Verification items for the finished model (mm, model axes). Face numbers are marked on the shaded views. Give positions to 0.01 mm unless a question says otherwise; leave off trailing zeros. Loops run counter-clockwise (first coordinate to the right, second up) from the corner with the lowest first, then second, coordinate; pieces in that order, holes last. Notation, with made-up numbers: M -11,16.25 L 8,16.25 A25 cw 8,40.25 Z; hole C 78,0.5 d3. An arc over 180 degrees is marked long. Answer in a Markdown table with one row per item.
```python
from build123d import *

# Parameters (mm, degrees)
ESBO_O1_W                  = 144
ESBO_O1_H                  = 74
ESBO_O1_W_2                = 140
ESBO_O1_H_2                = 70
RESSALTO_EXTRUS_O1_DEPTH   = 60
ESBO_O2_W                  = 144
ESBO_O2_H                  = 74
ESBO_O2_R                  = 2
RESSALTO_EXTRUS_O2_DEPTH   = 2
ESBO_O3_W                  = 14
ESBO_O3_H                  = 16
USB_FONTE_DEPTH            = 10
ESBO_O6_R                  = 1.65
ESBO_O6_W                  = 8
ESBO_O6_H                  = 35
SAIDA_DE_AR_DEPTH          = 1
SAIDA_DE_AR_DEPTH_BACK     = 75
ESBO_O7_W                  = 15
ESBO_O7_H                  = 30
DISPLAY_DEPTH              = 145
ESBO_O8_R                  = 4.5
ESBO_O8_R_2                = 1.35
RESSALTO_EXTRUS_O3_DEPTH   = 5
ESBO_O8_3_R                = 1.35
CORTE_EXTRUS_O4_DEPTH      = 3
ESBO_O9_R                  = 3
CORTE_EXTRUS_O5_DEPTH      = 2
CORTE_EXTRUS_O5_DEPTH_BACK = 10
RESSALTO_EXTRUS_O4_START   = -8
ESBO_O11_R                 = 1.65
RESSALTO_EXTRUS_O4_DEPTH   = 7
CORTE_EXTRUS_O6_DEPTH      = 3
ESBO_O13_R                 = 15.811388301
ESBO_O13_R_2               = 10
RESSALTO_EXTRUS_O5_DEPTH   = 2
ESBO_O13_3_R               = 10
CORTE_EXTRUS_O7_DEPTH      = 10
ESBO_O15_R                 = 22.5
ESBO_O15_R_2               = 1.6
CORTE_EXTRUS_O9_DEPTH      = 10
ESBO_O15_3_R               = 27.5
ESBO_O15_3_R_2             = 22.5
RESSALTO_EXTRUS_O6_DEPTH   = 2


with BuildPart() as part:
    # Esboço1 → Ressalto-extrusão1 (new body)
    with BuildSketch(Plane.XY):
        Rectangle(ESBO_O1_W, ESBO_O1_H)
        Rectangle(ESBO_O1_W_2, ESBO_O1_H_2, mode=Mode.SUBTRACT)
    extrude(amount=RESSALTO_EXTRUS_O1_DEPTH)

    # Esboço2 → Ressalto-extrusão2 (add)
    with BuildSketch(Plane(origin=(0, 0, 0), x_dir=(-1, 0, 0), z_dir=(0, 0, -1))):
        Rectangle(ESBO_O2_W, ESBO_O2_H)
        with Locations((-60, -27.5)):
            Circle(ESBO_O2_R, mode=Mode.SUBTRACT)
        with Locations((60, -27.5)):
            Circle(ESBO_O2_R, mode=Mode.SUBTRACT)
        with Locations((60, 27.5)):
            Circle(ESBO_O2_R, mode=Mode.SUBTRACT)
        with Locations((-60, 27.5)):
            Circle(ESBO_O2_R, mode=Mode.SUBTRACT)
    extrude(amount=-RESSALTO_EXTRUS_O2_DEPTH)

    # Esboço3 → USB + fonte (cut)
    with BuildSketch(Plane(origin=(72, 0, 0), x_dir=(0, 0, -1), z_dir=(1, 0, 0))):
        with Locations((-14, -17.1)):
            Rectangle(ESBO_O3_W, ESBO_O3_H)
    extrude(amount=-USB_FONTE_DEPTH, mode=Mode.SUBTRACT)

    # Esboço6 → saida de ar (cut, two sides)
    with BuildSketch(Plane.XZ.offset(37)) as saida_de_ar_sk:
        with Locations((-44, 50)):
            Circle(ESBO_O6_R)
        with Locations((44, 50)):
            Circle(ESBO_O6_R)
        with Locations((-58, 27.5)):
            Rectangle(ESBO_O6_W, ESBO_O6_H)
        with Locations((-45, 27.5)):
            Rectangle(ESBO_O6_W, ESBO_O6_H)
        with Locations((-32, 27.5)):
            Rectangle(ESBO_O6_W, ESBO_O6_H)
        with Locations((-19, 27.5)):
            Rectangle(ESBO_O6_W, ESBO_O6_H)
        with Locations((-6, 27.5)):
            Rectangle(ESBO_O6_W, ESBO_O6_H)
        with Locations((7, 27.5)):
            Rectangle(ESBO_O6_W, ESBO_O6_H)
        with Locations((20, 27.5)):
            Rectangle(ESBO_O6_W, ESBO_O6_H)
        with Locations((33, 27.5)):
            Rectangle(ESBO_O6_W, ESBO_O6_H)
        with Locations((46, 27.5)):
            Rectangle(ESBO_O6_W, ESBO_O6_H)
        with Locations((59, 27.5)):
            Rectangle(ESBO_O6_W, ESBO_O6_H)
    extrude(amount=SAIDA_DE_AR_DEPTH, mode=Mode.SUBTRACT)
    extrude(saida_de_ar_sk.sketch, amount=-SAIDA_DE_AR_DEPTH_BACK, mode=Mode.SUBTRACT)

    # Esboço7 → display (cut, through all)
    with BuildSketch(Plane.ZY.offset(72)):
        with Locations((52.5, 0)):
            Rectangle(ESBO_O7_W, ESBO_O7_H)
    extrude(amount=-DISPLAY_DEPTH, mode=Mode.SUBTRACT)

    # Esboço8 → Ressalto-extrusão3 (add)
    with BuildSketch(Plane(origin=(0, 0, 2), x_dir=(-1, 0, 0), z_dir=(0, 0, -1))):
        with Locations((32.3, 20.5)):
            Circle(ESBO_O8_R)
        with Locations((32.3, 20.5)):
            Circle(ESBO_O8_R_2, mode=Mode.SUBTRACT)
        with Locations((-50, 20.5)):
            Circle(ESBO_O8_R)
        with Locations((-50, 20.5)):
            Circle(ESBO_O8_R_2, mode=Mode.SUBTRACT)
        with Locations((-48.7, -27.67)):
            Circle(ESBO_O8_R)
        with Locations((-48.7, -27.67)):
            Circle(ESBO_O8_R_2, mode=Mode.SUBTRACT)
    extrude(amount=-RESSALTO_EXTRUS_O3_DEPTH)

    # Esboço8<3> → Corte-extrusão4 (cut, through all)
    with BuildSketch(Plane(origin=(0, 0, 2), x_dir=(-1, 0, 0), z_dir=(0, 0, -1))):
        with Locations((-48.7, -27.67)):
            Circle(ESBO_O8_3_R)
        with Locations((32.3, 20.5)):
            Circle(ESBO_O8_3_R)
        with Locations((-50, 20.5)):
            Circle(ESBO_O8_3_R)
    extrude(amount=CORTE_EXTRUS_O4_DEPTH, mode=Mode.SUBTRACT)

    # Esboço9 → Corte-extrusão5 (cut, two sides)
    with BuildSketch(Plane.XY.offset(2)) as corte_extrus_o5_sk:
        with Locations((50, 20.5)):
            Circle(ESBO_O9_R)
        with Locations((48.7, -27.67)):
            Circle(ESBO_O9_R)
        with Locations((-32.3, 20.5)):
            Circle(ESBO_O9_R)
    extrude(amount=CORTE_EXTRUS_O5_DEPTH, mode=Mode.SUBTRACT)
    extrude(corte_extrus_o5_sk.sketch, amount=-CORTE_EXTRUS_O5_DEPTH_BACK, mode=Mode.SUBTRACT)

    # Esboço11 → Ressalto-extrusão4 (add)
    with BuildSketch(Plane.XY.offset(60).offset(RESSALTO_EXTRUS_O4_START)):
        with BuildLine():
            Line((70, -25), (65, -25))
            ThreePointArc((65, -25), (60, -20), (65, -15))
            Line((65, -15), (70, -15))
            Line((70, -15), (70, -25))
        make_face()
        with Locations((65, -20)):
            Circle(ESBO_O11_R, mode=Mode.SUBTRACT)
        with BuildLine():
            Line((70, 35), (65, 35))
            ThreePointArc((65, 35), (61.464466094, 26.464466094), (70, 30))
            Line((70, 30), (70, 35))
        make_face()
        with Locations((65, 30)):
            Circle(ESBO_O11_R, mode=Mode.SUBTRACT)
        with BuildLine():
            Line((-70, -25), (-70, -15))
            Line((-70, -15), (-65, -15))
            ThreePointArc((-65, -15), (-60, -20), (-65, -25))
            Line((-65, -25), (-70, -25))
        make_face()
        with Locations((-65, -20)):
            Circle(ESBO_O11_R, mode=Mode.SUBTRACT)
        with BuildLine():
            Line((-65, 35), (-70, 35))
            Line((-70, 35), (-70, 30))
            ThreePointArc((-70, 30), (-61.464466094, 26.464466094), (-65, 35))
        make_face()
        with Locations((-65, 30)):
            Circle(ESBO_O11_R, mode=Mode.SUBTRACT)
    extrude(amount=-RESSALTO_EXTRUS_O4_DEPTH)

    # Esboço12 → Corte-extrusão6 (cut)
    with BuildSketch(Plane(origin=(0, 0, 45), x_dir=(-1, 0, 0), z_dir=(0, 0, -1))):
        Polygon((-61.824573519, 30), (-63.41228676, 32.75), (-66.58771324, 32.75), (-68.175426481, 30), (-66.58771324, 27.25), (-63.41228676, 27.25), align=None)
        Polygon((61.824573519, 30), (63.41228676, 27.25), (66.58771324, 27.25), (68.175426481, 30), (66.58771324, 32.75), (63.41228676, 32.75), align=None)
        Polygon((-61.824573519, -20), (-63.41228676, -17.25), (-66.58771324, -17.25), (-68.175426481, -20), (-66.58771324, -22.75), (-63.41228676, -22.75), align=None)
        Polygon((61.824573519, -20), (63.41228676, -22.75), (66.58771324, -22.75), (68.175426481, -20), (66.58771324, -17.25), (63.41228676, -17.25), align=None)
    extrude(amount=-CORTE_EXTRUS_O6_DEPTH, mode=Mode.SUBTRACT)

    # Esboço13 → Ressalto-extrusão5 (add)
    with BuildSketch(Plane(origin=(0, 37, 0), x_dir=(1, 0, 0), z_dir=(0, 1, 0))):
        with Locations((29, -25)):
            Circle(ESBO_O13_R)
        with Locations((29, -25)):
            Circle(ESBO_O13_R_2, mode=Mode.SUBTRACT)
    extrude(amount=-RESSALTO_EXTRUS_O5_DEPTH)

    # Esboço13<3> → Corte-extrusão7 (cut)
    with BuildSketch(Plane(origin=(0, 37, 0), x_dir=(1, 0, 0), z_dir=(0, 1, 0))):
        with Locations((29, -25)):
            Circle(ESBO_O13_3_R)
    extrude(amount=-CORTE_EXTRUS_O7_DEPTH, mode=Mode.SUBTRACT)

    # Esboço15 → Corte-extrusão9 (cut)
    with BuildSketch(Plane(origin=(0, 37, 0), x_dir=(1, 0, 0), z_dir=(0, 1, 0))):
        with Locations((-16, -31)):
            Circle(ESBO_O15_R)
        with Locations((-41, -56)):
            Circle(ESBO_O15_R_2)
        with Locations((9, -56)):
            Circle(ESBO_O15_R_2)
        with Locations((-41, -6)):
            Circle(ESBO_O15_R_2)
        with Locations((9, -6)):
            Circle(ESBO_O15_R_2)
    extrude(amount=-CORTE_EXTRUS_O9_DEPTH, mode=Mode.SUBTRACT)

    # Esboço15<3> → Ressalto-extrusão6 (add)
    with BuildSketch(Plane(origin=(0, 37, 0), x_dir=(1, 0, 0), z_dir=(0, 1, 0))):
        with Locations((-16, -31)):
            Circle(ESBO_O15_3_R)
        with Locations((-16, -31)):
            Circle(ESBO_O15_3_R_2, mode=Mode.SUBTRACT)
    extrude(amount=-RESSALTO_EXTRUS_O6_DEPTH)


solid = part.part
```
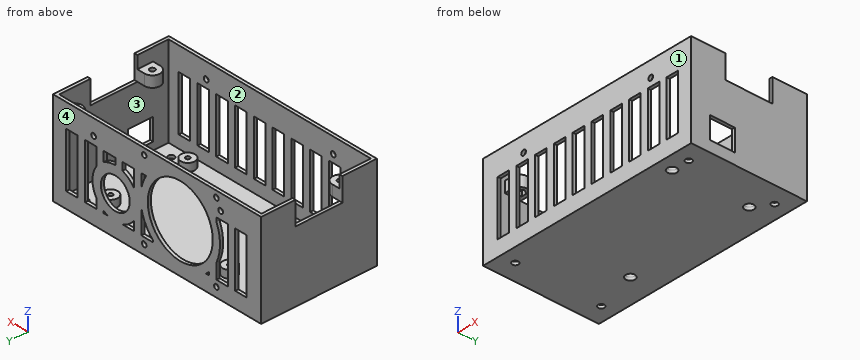
Item 1: Sectioned sample at C-C (y = 12.5). Record the cut outline in (x, z).
Reported:
| item | result |
|---|---|
| outline | M -72,0 L 72,0 L 72,45 L 70,45 L 70,2 L -70,2 L -70,45 L -72,45 Z |
Item 2: Release check for a two-part mould opening along Y. For the marked faces 1, 2, 3 and 4 record: released by +Y, released by -Y, zero draft, split by the parting line, or undercut.
Reported:
| item | result |
|---|---|
| face 1 | released by -Y |
| face 2 | undercut |
| face 3 | undercut |
| face 4 | released by +Y |
Item 3: Sectioned sample at B-B (x = 40.5). Record the cut outline in (y, z), and give its area (3 significant figures).
Reported:
| item | result |
|---|---|
| outline | M -37,0 L 37,0 L 37,60 L 35,60 L 35,2 L -35,2 L -35,60 L -37,60 Z |
| area | 380 mm^2 |
Item 4: Sectioned sample at A-A (y = -12.5). Record the cut outline in (x, z), and give its area (3 significant figures).
Reported:
| item | result |
|---|---|
| outline | M -72,0 L 72,0 L 72,7 L 70,7 L 70,2 L -70,2 L -70,45 L -72,45 Z; M 70,21 L 72,21 L 72,45 L 70,45 Z |
| area | 432 mm^2 |
Item 5: Go/stop test with flat-tipped pins: pin 1 (4.5 mm diameter, centred on x = -65, y = -20, fed in from +Z); pin 2 (4 mm diameter, centred on x = 44.5, y = -28, fed in from +Z); pin 3 (5 mm diameter, centred on x = -41.5, y = 20, fed in from +Z). Record where each tip stops, or that it passes through.
Reported:
| item | result |
|---|---|
| pin 1 | stops at z = 52 |
| pin 2 | stops at z = 7 |
| pin 3 | stops at z = 2 |
Item 6: Scan lines: L1, parallel to X at y = 36.35, z = 6; L2, parallel to X at y = 25, z = 35; L3, parallel to Y at x = -3, z = 50. Record each from-to range of solid material in increasing order. Write a range as [from, to].
Reported:
| item | result |
|---|---|
| L1 | x = [-72, -42.6], [-39.4, 7.4], [10.6, 72] |
| L2 | x = [-72, -70], [70, 72] |
| L3 | y = [-37, -35], [35, 37] |
